Geometry: final body of the model. Coordinates: model frame, mm. A direction names the side the tool comes from. Give positions to 0.01 mm unless a question says otherwise; leave off trailing zeros. Loops run counter-clockwise (first coordinate to the right, second up) from the corner with the lowest first, then second, coordinate; pieces in that order, holes last. Notation, with made-up numbers: (-17.5, 15) - (-8.5, 15) arc R21 ccw to (-8.5, 26) - close; hole circle Ø8 at (32, -26). An arc over 180 degrees is marked (long way). Answer in a Markdown table with one row per item.
from build123d import *

# Parameters (mm, degrees)
SKETCH1_R         = 2.3241
EXTRUDE1_DEPTH    = 28.2448
SKETCH3_OUTSIDE_W = 12.448
SKETCH3_OUTSIDE_H = 12.448
SKETCH3_OUTSIDE_R = 1.4732
EXTRUDE2_DEPTH    = 25.4
EXTRUDE3_DEPTH    = 1.778


with BuildPart() as part:
    # Sketch1 → Extrude1 (new body)
    with BuildSketch(Plane.XY):
        Circle(SKETCH1_R)
    extrude(amount=EXTRUDE1_DEPTH)

    # Sketch3 outside → Extrude2 (cut)
    with BuildSketch(Plane(origin=(0, 0, 0), x_dir=(-1, 0, 0), z_dir=(0, 0, -1))):
        Rectangle(SKETCH3_OUTSIDE_W, SKETCH3_OUTSIDE_H)
        Circle(SKETCH3_OUTSIDE_R, mode=Mode.SUBTRACT)
    extrude(amount=-EXTRUDE2_DEPTH, mode=Mode.SUBTRACT)

    # Sketch4 → Extrude3 (cut)
    with BuildSketch(Plane.XY.offset(28.2448)):
        Polygon((1.466469684, 0), (0.733234842, 1.27), (-0.733234842, 1.27), (-1.466469684, 0), (-0.733234842, -1.27), (0.733234842, -1.27), align=None)
    extrude(amount=-EXTRUDE3_DEPTH, mode=Mode.SUBTRACT)


solid = part.part
Q1. Cut plane C-C (z = 7.5). Output: boundary loops of the cut face in (x, y), and give its area (3 significant figures).
Check values:
| item | result |
|---|---|
| outline | circle Ø2.95 at (0, 0) |
| area | 6.82 mm² |
Q2. Reachability of faces 1 (the cylindrical face through (-1.405, 0.443, 12.522)), 2 (the flat face through (0, 0, 0)), 3 (the flat face through (0, -1.27, 27)) from +Z, -Z, +X, -X, +Y, -Y: full face, straight path, thin tool, end or side. Return the list, or none.
Check values:
| item | result |
|---|---|
| face 1 | -Z |
| face 2 | -Z, +X, -X, +Y, -Y |
| face 3 | +Z |
Q3. First-contact query: pin 1 (1 mm diameter, centred on y = 0, z = 11, fed in from -X); pin 2 (2 mm diameter, centred on y = 1.5, z = 15, fed in from -X); pin 3 (1.5 mm diameter, centred on y = -1.5, z = 22, fed in from +X). Flat tips, straight axial feed; report the tip coordinate or a pass-through.
Check values:
| item | result |
|---|---|
| pin 1 | x = -1.47 |
| pin 2 | x = -1.39 |
| pin 3 | x = 1.27 |
Q4. Cut plane B-B (y = -0.35). Output: boundary loops of the cut face in (x, z).
Check values:
| item | result |
|---|---|
| outline | (-2.3, 25.4) - (-1.43, 25.4) - (-1.43, 0) - (1.43, 0) - (1.43, 25.4) - (2.3, 25.4) - (2.3, 28.24) - (1.26, 28.24) - (1.26, 26.47) - (-1.26, 26.47) - (-1.26, 28.24) - (-2.3, 28.24) - close |
Q5. Material intervals for line 1 along Z through (x, y) = (-1.7, 1.3); line 2 along Z through (x, y) = (-1.05, 0.5); line 3 along X through (y, z) = (0.6, 27), sorted ascending.
Check values:
| item | result |
|---|---|
| line 1 | 25.4 to 28.24 |
| line 2 | 0 to 26.47 |
| line 3 | -2.25 to -1.12, 1.12 to 2.25 |
Q6. Cut plane A-A (x = 0). Output: boundary loops of the cut face in (y, z), and give its area (3 significant figures).
Check values:
| item | result |
|---|---|
| outline | (-2.32, 25.4) - (-1.47, 25.4) - (-1.47, 0) - (1.47, 0) - (1.47, 25.4) - (2.32, 25.4) - (2.32, 28.24) - (1.27, 28.24) - (1.27, 26.47) - (-1.27, 26.47) - (-1.27, 28.24) - (-2.32, 28.24) - close |
| area | 83.5 mm² |
Q7. Cut plane D-D (y = -1.75). Output: boundary loops of the cut face in (x, z), and give its area (3 significant figures).
Check values:
| item | result |
|---|---|
| outline | (-1.53, 25.4) - (1.53, 25.4) - (1.53, 28.24) - (-1.53, 28.24) - close |
| area | 8.70 mm² |
Q8. Draft query along X for faces 4 (the cylindrical face through (-0.5, -2.27, 26.8)), 5 (the flat face through (0, -2, 25.4)), 6 (the flat face through (1.105, 0.626, 27.368)). Return one class per face: pulls with the +X half, pulls with the -X half, needs draft (parallel to the pull), parting line crosses it, or undercut.
Check values:
| item | result |
|---|---|
| face 4 | parting line crosses it |
| face 5 | needs draft |
| face 6 | undercut |
